Geometry: see drawing. Coordinates: mm, zero at the bounding-box minimum. Coordinates: 2 decimals unless noted, no trailing zeros. Loops run counter-clockwise (first coordinate to the right, second up) from the corner with the lowest first, then second, coordinate; pieces in that order, holes last. Notation, with made-up numbers: (-10, -12) - (19, -12) arc R8 ccw to (19, -7) - close; hole circle Ø6 at (84.5, 4.5). An arc over 180 degrees is marked (long way). Answer in a Markdown table with one row per item.
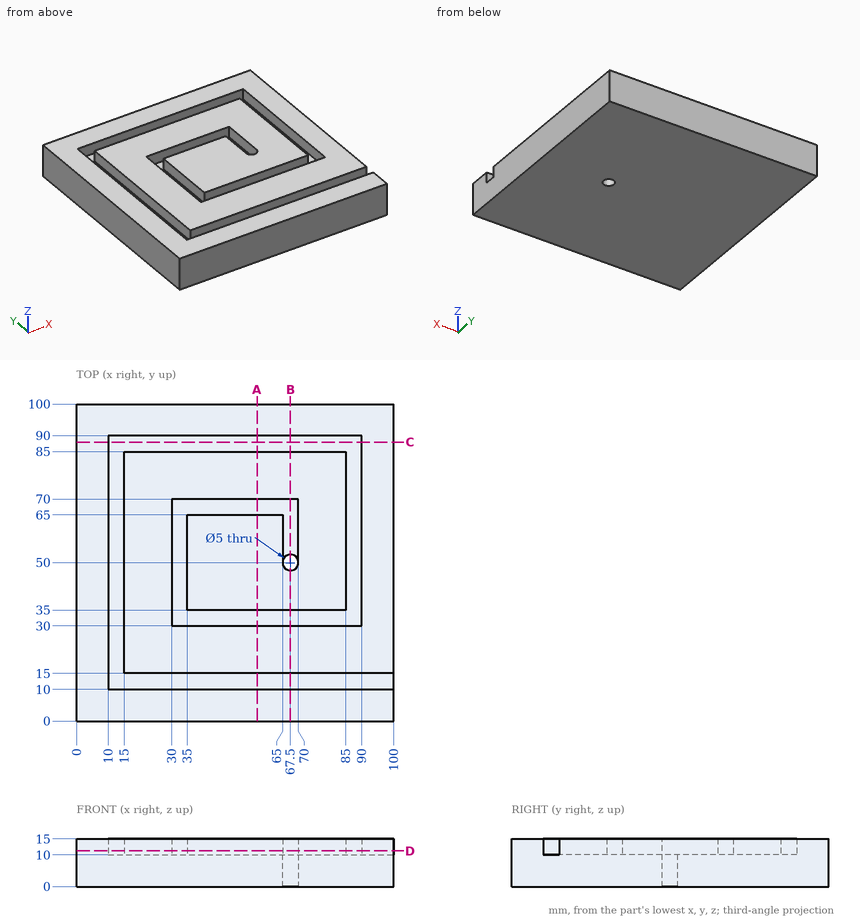
(1) Ray query, probe 1 along Y at (x, z) = (67.5, 12); probe 2 along Y at (x, z) = (21, 10.5); probe 3 along X at (y, z) = (50, 7.25). Return the intervals inside material, ascending.
Verdict:
| item | result |
|---|---|
| probe 1 | y = 0 to 10, 15 to 30, 35 to 47.5, 70 to 85, 90 to 100 |
| probe 2 | y = 0 to 10, 15 to 85, 90 to 100 |
| probe 3 | x = 0 to 65, 70 to 100 |
(2) Cut plane A-A on x = 57. Output: boundary loops of the cut face in (y, z), then the cut area to 3 significant figures.
Verdict:
| item | result |
|---|---|
| outline | (0, 0) - (100, 0) - (100, 15) - (90, 15) - (90, 10) - (85, 10) - (85, 15) - (70, 15) - (70, 10) - (65, 10) - (65, 15) - (35, 15) - (35, 10) - (30, 10) - (30, 15) - (15, 15) - (15, 10) - (10, 10) - (10, 15) - (0, 15) - close |
| area | 1,400 mm² |
(3) Cut plane D-D on z = 11.25. Output: boundary loops of the cut face in (x, y), then the cut area to 3 significant figures.
Verdict:
| item | result |
|---|---|
| outline | (0, 0) - (100, 0) - (100, 10) - (10, 10) - (10, 90) - (90, 90) - (90, 30) - (30, 30) - (30, 70) - (70, 70) - (70, 50) arc R2.5 cw to (65, 50) - (65, 65) - (35, 65) - (35, 35) - (85, 35) - (85, 85) - (15, 85) - (15, 15) - (100, 15) - (100, 100) - (0, 100) - close |
| area | 7,820 mm² |
(4) Cut plane C-C on y = 88. Output: boundary loops of the cut face in (x, z).
Verdict:
| item | result |
|---|---|
| outline | (0, 0) - (100, 0) - (100, 15) - (90, 15) - (90, 10) - (10, 10) - (10, 15) - (0, 15) - close |
(5) Cut plane B-B on x = 67.5. Output: boundary loops of the cut face in (y, z), then the cut area to 3 significant figures.
Verdict:
| item | result |
|---|---|
| outline | (0, 0) - (47.5, 0) - (47.5, 15) - (35, 15) - (35, 10) - (30, 10) - (30, 15) - (15, 15) - (15, 10) - (10, 10) - (10, 15) - (0, 15) - close; (52.5, 0) - (100, 0) - (100, 15) - (90, 15) - (90, 10) - (85, 10) - (85, 15) - (70, 15) - (70, 10) - (52.5, 10) - close |
| area | 1,260 mm² |
(6) First-contact query: pin 1 Ø3 at (x, y) = (67.5, 50) entering from -Z. Flat tip, straight axial feed; report the tip coordinate or a pass-through.
Verdict:
| item | result |
|---|---|
| pin 1 | passes through |
